Read the model definition and answer for the solid it produces. Units are mm, in the model's axes. A direction names the side the tool comes from. Coordinates: 2 decimals unless noted, no trailing zeros. Order: outer loops, then holes, each group sorted by start corner. A loop starts at its lowest first (then second) coordinate and runs counter-clockwise, first axis right, second up. Notation, with made-up numbers: M -4,73.25 L 44,73.25 A16 cw 44,104.25 Z; hole C 31,22.5 d8. An arc over 180 degrees is marked long. One line per question, with ' | ' between items. Start each with the question number.
1) Find section C-C, the plane y = 4.4. Write down the section's boundary in (x, z), plus the area to 3 significant figures.
2) Given P1, Ø2, axis at x = -5.5, y = 2.5, coming from the -Z side; P2, Ø4.5, axis at x = -0.5, z = 0, coming from the -Y side, each flat-ended and moving along its own axis, determine where each tip first touches the part or whether it passes through.
3) A tool of negligible diameter and unlimited length cuts with its end or side. For faces 4 (the face through (-0.37, 4.01, 1.66)), 5 (the face through (0, 1, -2.85)), from which of +Z, -Z, +X, -X, +Y, -Y can it reach the whole face along a straight path? Write none if from no direction.
4) The mould has two halves that part along X. Classify faces 1 (the face through (-2.46, 1.48, 1.44)), 2 (the face through (8, 3, 0)), 3 (the face through (-3, 0, 1)): +X half, -X half, draft (parallel to the pull), parting line (faces both ways), or undercut.
5) Consider probe 1 along X at (y, z) = (3.5, 0); probe 2 along Z at (x, y) = (1, 1.55); probe 3 along Y at (x, z) = (2.5, 0.25). Determine where each line is inside the solid, lowest interval first.
6) Find section D-D, the plane x = -3. Write down the section's boundary in (y, z).
7) Find section B-B, the plane y = 2.6. Write down the section's boundary in (x, z), plus the area to 3 significant figures.
8) Find section A-A, the plane x = 0. Write down the section's boundary in (y, z).
from build123d import *

# Parameters (mm, degrees)
BOSS_EXTRU_1_DEPTH = 5
ESQUISSE2_R        = 1.7
BOSS_EXTRU_2_DEPTH = 2
CONG_1_R           = 1


with BuildPart() as part:
    # Esquisse1 → Boss.-Extru.1 (new body)
    with BuildSketch(Plane(origin=(0, 0, 0), x_dir=(1, 0, 0), z_dir=(0, 1, 0))):
        with BuildLine():
            Line((-4, 4), (4, 4))
            ThreePointArc((4, 4), (8, 0), (4, -4))
            Line((4, -4), (-4, -4))
            ThreePointArc((-4, -4), (-8, 0), (-4, 4))
        make_face()
        Polygon((-1.645448267, 2.85), (1.645448267, 2.85), (3.290896534, 0), (1.645448267, -2.85), (-1.645448267, -2.85), (-3.290896534, 0), align=None, mode=Mode.SUBTRACT)
    extrude(amount=BOSS_EXTRU_1_DEPTH)

    # Esquisse2 → Boss.-Extru.2 (add)
    with BuildSketch(Plane(origin=(0, 5, 0), x_dir=(1, 0, 0), z_dir=(0, 1, 0))):
        with BuildLine():
            Line((-4, -4), (4, -4))
            ThreePointArc((4, -4), (8, 0), (4, 4))
            Line((4, 4), (-4, 4))
            ThreePointArc((-4, 4), (-8, 0), (-4, -4))
        make_face()
        Circle(ESQUISSE2_R, mode=Mode.SUBTRACT)
    extrude(amount=-BOSS_EXTRU_2_DEPTH)

    # Congé1
    cong_1_edges = [part.edges().sort_by_distance(p)[0] for p in [
        (0, 0, -4),
        (8, 0, 0),
        (0, 0, 4),
        (-8, 0, 0),
    ]]
    fillet(cong_1_edges, radius=CONG_1_R)


solid = part.part
Report:
1) outline: M -4,-4 L 4,-4 A4 ccw 4,4 L -4,4 A4 ccw Z; hole C 0,0 d3.4 | area: 105 mm^2
2) P1: stops at z = -3.97 | P2: stops at y = 3
3) face 4: +Y, -Y | face 5: -Y
4) face 1: undercut | face 2: +X half | face 3: draft
5) probe 1: x = -8 to -1.7, 1.7 to 8 | probe 2: z = -4 to -2.85, 2.85 to 4 | probe 3: y = 3 to 5
6) outline: M 0,-3 A1 ccw 1,-4 L 5,-4 L 5,4 L 1,4 A1 ccw 0,3 L 0,0.5 L 3,0.5 L 3,-0.5 L 0,-0.5 Z
7) outline: M -4,-4 L 4,-4 A4 ccw 4,4 L -4,4 A4 ccw Z; hole M -3.29,0 L -1.65,-2.85 L 1.65,-2.85 L 3.29,0 L 1.65,2.85 L -1.65,2.85 Z | area: 86.1 mm^2
8) outline: M 0,-3 A1 ccw 1,-4 L 5,-4 L 5,-1.7 L 3,-1.7 L 3,-2.85 L 0,-2.85 Z; M 0,2.85 L 3,2.85 L 3,1.7 L 5,1.7 L 5,4 L 1,4 A1 ccw 0,3 Z
